from build123d import *

# Parameters (mm, degrees)
SKETCH1_R           = 5
SKETCH1_R_2         = 4.435
BOSS_EXTRUDE1_DEPTH = 5


with BuildPart() as part:
    # Sketch1 → Boss-Extrude1 (new, symmetric)
    with BuildSketch(Plane.XY):
        with BuildLine():
            Line((36.66060556, 16), (0, 16))
            ThreePointArc((0, 16), (-16, 0), (0, -16))
            Line((0, -16), (36.66060556, -16))
            ThreePointArc((36.66060556, -16), (-3.354853263, -39.859063707), (-38.819261012, -9.647018944))
            ThreePointArc((-38.819261012, -9.647018944), (-39.173778039, -9.100420505), (-39.789742537, -8.888194417))
            Line((-39.789742537, -8.888194417), (-214, -8.888194417))
            ThreePointArc((-214, -8.888194417), (-222.888194417, 0), (-214, 8.888194417))
            Line((-214, 8.888194417), (-39.789742537, 8.888194417))
            ThreePointArc((-39.789742537, 8.888194417), (-39.173778039, 9.100420505), (-38.819261012, 9.647018944))
            ThreePointArc((-38.819261012, 9.647018944), (-3.354853263, 39.859063707), (36.66060556, 16))
        make_face()
        with Locations((0, 27.5)):
            Circle(SKETCH1_R, mode=Mode.SUBTRACT)
        with Locations((-28, 0)):
            Circle(SKETCH1_R, mode=Mode.SUBTRACT)
        with Locations((0, -27.5)):
            Circle(SKETCH1_R, mode=Mode.SUBTRACT)
        with Locations((-214, 0)):
            Circle(SKETCH1_R_2, mode=Mode.SUBTRACT)
        with BuildLine():
            Line((-188, 3), (-58, 3))
            ThreePointArc((-58, 3), (-55, 0), (-58, -3))
            Line((-58, -3), (-188, -3))
            ThreePointArc((-188, -3), (-191, 0), (-188, 3))
        make_face(mode=Mode.SUBTRACT)
    extrude(amount=BOSS_EXTRUDE1_DEPTH, both=True)


solid = part.part
Verification items for the finished model (mm, model axes). A direction names the side the tool comes from. Round coordinates to 2 decimals unless told otherwise and drop trailing zeros. Write each loop counter-clockwise with the first axis right and the second up, starting at its lowest first coordinate (ties: lowest second). Pieces come first, ordered by that corner, then holes.
(1) Mould release check, pull along Y, two halves, no side actions. Record for faces 1 (the cylindrical face through (-191, 0, 0)), 2 (the cylindrical face through (-222.886, -0.195, 0.07)), 3 (the cylindrical face through (-4, 39.8, 0.1)): pulls with the +Y half, pulls with the -Y half, needs draft (parallel to the pull), parting line crosses it, or undercut.
Returned:
face 1: undercut
face 2: parting line crosses it
face 3: pulls with the +Y half
(2) Section check A-A (y = 0). Enter the section's corners in (x, z) (3 decimals).
Returned:
outline: (-222.888, -5) - (-218.435, -5) - (-218.435, 5) - (-222.888, 5) - close; (-209.565, -5) - (-191, -5) - (-191, 5) - (-209.565, 5) - close; (-55, -5) - (-33, -5) - (-33, 5) - (-55, 5) - close; (-23, -5) - (-16, -5) - (-16, 5) - (-23, 5) - close
(3) Depth check by flat-ended pin: pin 1 Ø1 at (y, z) = (-27, 2) entering from -X; pin 2 Ø1.5 at (x, z) = (-129.5, 2) entering from +Y; pin 3 Ø3 at (x, z) = (-70.5, -1) entering from -Y; pin 4 Ø9 at (x, y) = (0, 27.5) entering from +Z. Enter the tip coordinate at first touch or a pass-through.
Returned:
pin 1: stops at x = -29.96
pin 2: stops at y = 8.89
pin 3: stops at y = -8.89
pin 4: passes through
(4) Section check C-C (x = -92.5). Enter the section's corners in (y, z).
Returned:
outline: (-8.89, -5) - (-3, -5) - (-3, 5) - (-8.89, 5) - close; (3, -5) - (8.89, -5) - (8.89, 5) - (3, 5) - close
(5) Material ranges on line 1 (Y direction, x = 0, z = -2); line 2 (X direction, y = 0.5, z = 3.75); line 3 (Y direction, x = -113.5, z = -2), recorded low to high.
Returned:
line 1: y = -40 to -32.5, -22.5 to -16, 16 to 22.5, 32.5 to 40
line 2: x = -222.87 to -218.41, -209.59 to -190.96, -55.04 to -32.97, -23.03 to -15.99
line 3: y = -8.89 to -3, 3 to 8.89
(6) Section check D-D (y = 27.5). Enter the section's corners in (x, z), plus the area to 3 significant figures.
Returned:
outline: (-29.05, -5) - (-5, -5) - (-5, 5) - (-29.05, 5) - close; (5, -5) - (29.05, -5) - (29.05, 5) - (5, 5) - close
area: 481 mm2
(7) Section check B-B (z = -0.75). Enter the section's corners in (x, y) (3 decimals), plus the area to 3 significant figures.
Returned:
outline: (-214, -8.888) - (-39.79, -8.888) arc R1 cw to (-38.819, -9.647) arc R40 ccw to (36.661, -16) - (0, -16) arc R16 cw to (0, 16) - (36.661, 16) arc R40 ccw to (-38.819, 9.647) arc R1 cw to (-39.79, 8.888) - (-214, 8.888) arc R8.888 ccw to start; hole circle Ø8.87 at (-214, 0); hole (-188, -3) - (-58, -3) arc R3 ccw to (-58, 3) - (-188, 3) arc R3 ccw to start; hole circle Ø10 at (-28, 0); hole circle Ø10 at (0, -27.5); hole circle Ø10 at (0, 27.5)
area: 5,500 mm2
(8) Access from +Z, -Z, +X, -X, +Y, -Y to the whole of each face (thin tool, end or side, straight path). Record for faces 4 (the flat face through (19, 16, 0)), 5 (the flat face through (-124, 3, 0)), 6 (the flat face through (-126, -8.888, 0)).
Returned:
face 4: +Z, -Z, +X
face 5: +Z, -Z
face 6: +Z, -Z, -X, -Y
